Design review of the part built by this model. Coordinates are the model's own, in mm. Face numbers are marked on the shaded views. A direction names the side the tool comes from. Coordinates: 2 decimals unless noted, no trailing zeros. Order: outer loops, then holes, each group sorted by start corner. A loop starts at its lowest first (then second) coordinate and runs counter-clockwise, first axis right, second up. Notation, with made-up numbers: (38, 44) - (77, 44) arc R21 cw to (77, 66) - close; hole circle Ø5 at (84.5, 6). An arc over 180 degrees is marked (long way). Write item = value, one per line. Start each with the question number.
```python
from build123d import *

# Parameters (mm, degrees)
SKETCH1_R               = 11
SKETCH1_R_2             = 1
BOSS_EXTRUDE1_DEPTH     = 2
SKETCH2_R               = 4
CUT_EXTRUDE1_DEPTH      = 16.684387141
SKETCH4_W               = 1.5
SKETCH4_H               = 3
CUT_EXTRUDE3_DEPTH      = 4
BOSS_EXTRUDE2_START     = 20
SKETCH5_R               = 6
SKETCH5_R_2             = 4
BOSS_EXTRUDE2_DEPTH     = 20
BOSS_EXTRUDE3_START     = 20
SKETCH6_R               = 6
BOSS_EXTRUDE3_DEPTH     = 20
CUT_EXTRUDE4_DEPTH      = 5
CUT_EXTRUDE4_DEPTH_BACK = 1
SKETCH7_R               = 1
SKETCH8_R               = 2
CUT_EXTRUDE5_DEPTH      = 1


with BuildPart() as part:
    # Sketch1 → Boss-Extrude1 (new body)
    with BuildSketch(Plane(origin=(0, 0, 0), x_dir=(1, 0, 0), z_dir=(0, 1, 0))):
        with Locations(Location((0, 0, 0), (0, 0, 270))):
            Circle(SKETCH1_R)
        with Locations(Location((0, 8, 0), (0, 0, 270))):
            Circle(SKETCH1_R_2, mode=Mode.SUBTRACT)
        with Locations(Location((5.656854249, 5.656854249, 0), (0, 0, 270))):
            Circle(SKETCH1_R_2, mode=Mode.SUBTRACT)
        with Locations(Location((8, 0, 0), (0, 0, 270))):
            Circle(SKETCH1_R_2, mode=Mode.SUBTRACT)
        with Locations(Location((5.656854249, -5.656854249, 0), (0, 0, 270))):
            Circle(SKETCH1_R_2, mode=Mode.SUBTRACT)
        with Locations(Location((0, -8, 0), (0, 0, 270))):
            Circle(SKETCH1_R_2, mode=Mode.SUBTRACT)
        with Locations(Location((-5.656854249, -5.656854249, 0), (0, 0, 270))):
            Circle(SKETCH1_R_2, mode=Mode.SUBTRACT)
        with Locations(Location((-8, 0, 0), (0, 0, 270))):
            Circle(SKETCH1_R_2, mode=Mode.SUBTRACT)
        with Locations(Location((-5.656854249, 5.656854249, 0), (0, 0, 270))):
            Circle(SKETCH1_R_2, mode=Mode.SUBTRACT)
    extrude(amount=BOSS_EXTRUDE1_DEPTH)

    # Sketch2 → Cut-Extrude1 (cut, through all)
    with BuildSketch(Plane(origin=(0, 2, 0), x_dir=(1, 0, 0), z_dir=(0, 1, 0))):
        with Locations(Location((0, 0, 0), (0, 0, 270))):
            Circle(SKETCH2_R)
    extrude(amount=-CUT_EXTRUDE1_DEPTH, mode=Mode.SUBTRACT)

    # Sketch4 → Cut-Extrude3 (cut)
    with BuildSketch(Plane(origin=(0, 2, 0), x_dir=(1, 0, 0), z_dir=(0, 1, 0))):
        with Locations((0, 11)):
            Rectangle(SKETCH4_W, SKETCH4_H)
    extrude(amount=-CUT_EXTRUDE3_DEPTH, mode=Mode.SUBTRACT)

    # Sketch5 → Boss-Extrude2 (add)
    with BuildSketch(Plane(origin=(0, 2, 0), x_dir=(1, 0, 0), z_dir=(0, 1, 0)).offset(BOSS_EXTRUDE2_START)):
        with Locations(Location((0, 0, 0), (0, 0, 270))):
            Circle(SKETCH5_R)
        with Locations(Location((0, 0, 0), (0, 0, 270))):
            Circle(SKETCH5_R_2, mode=Mode.SUBTRACT)
    extrude(amount=-BOSS_EXTRUDE2_DEPTH)

    # Sketch6 → Boss-Extrude3 (add)
    with BuildSketch(Plane(origin=(0, 22, 0), x_dir=(1, 0, 0), z_dir=(0, 1, 0)).offset(BOSS_EXTRUDE3_START)):
        with Locations(Location((0, 0, 0), (0, 0, 270))):
            Circle(SKETCH6_R)
        with BuildLine():
            ThreePointArc((-0.967204218, 0.254), (-0.707472278, 0.706741095), (-0.255, 0.966941053))
            Line((-0.255, 0.966941053), (-0.255, 1.476941053))
            Line((-0.255, 1.476941053), (0.255, 1.476941053))
            Line((0.255, 1.476941053), (0.255, 0.966941053))
            ThreePointArc((0.255, 0.966941053), (0.707472278, 0.706741095), (0.967204218, 0.254))
            Line((0.967204218, 0.254), (1.475204218, 0.254))
            Line((1.475204218, 0.254), (1.475204218, -0.254))
            Line((1.475204218, -0.254), (0.967204218, -0.254))
            ThreePointArc((0.967204218, -0.254), (0.707106781, -0.707106781), (0.254, -0.967204218))
            Line((0.254, -0.967204218), (0.254, -1.475204218))
            Line((0.254, -1.475204218), (-0.254, -1.475204218))
            Line((-0.254, -1.475204218), (-0.254, -0.967204218))
            ThreePointArc((-0.254, -0.967204218), (-0.707106781, -0.707106781), (-0.967204218, -0.254))
            Line((-0.967204218, -0.254), (-1.475204218, -0.254))
            Line((-1.475204218, -0.254), (-1.475204218, 0.254))
            Line((-1.475204218, 0.254), (-0.967204218, 0.254))
        make_face(mode=Mode.SUBTRACT)
    extrude(amount=-BOSS_EXTRUDE3_DEPTH)

    # Sketch7 → Cut-Extrude4 (cut, two sides: drawn at the far end of the back side and taken through both)
    with BuildSketch(Plane.XY.offset(-CUT_EXTRUDE4_DEPTH_BACK)):
        with Locations(Location((0, 35, 0), (0, 0, 165.285661458))):
            Circle(SKETCH7_R)
    extrude(amount=CUT_EXTRUDE4_DEPTH + CUT_EXTRUDE4_DEPTH_BACK, mode=Mode.SUBTRACT)

    # Sketch8 → Cut-Extrude5 (cut)
    with BuildSketch(Plane.XY.offset(6)):
        with Locations((0, 35)):
            Circle(SKETCH8_R)
    extrude(amount=-CUT_EXTRUDE5_DEPTH, mode=Mode.SUBTRACT)


solid = part.part
```
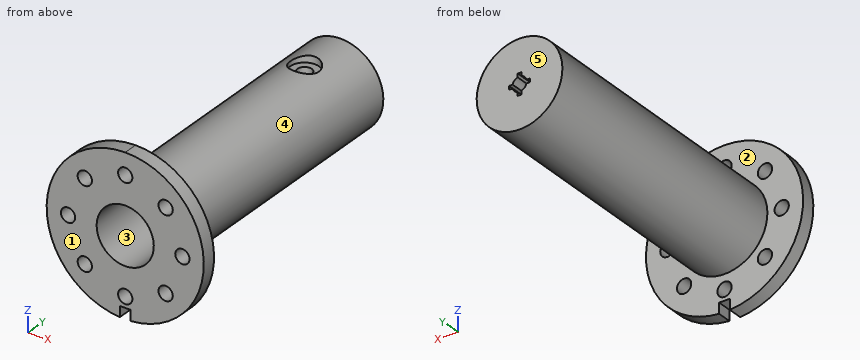
Item 1: Add section C-C on z = 2.75. Give the boundary of the cut face in (x, y), plus the area to 3 significant figures.
Item 2: Mouldability with a two-part tool opening along Z and no side actions: class the marked faces 3, 4 and 5 as +Z half, -Z half, draft (parallel to the pull), parting line (faces both ways), or undercut.
Item 3: For line 1 (X direction, y = 12.5, z = 0); line 2 (Y direction, x = -2.5, z = 8.75); line 3 (Y direction, x = -2.5, z = 1.75), list the stretches that pass through material, from the lowest coordinate up.
Item 4: Add section A-A on z = -8. Give the boundary of the cut face in (x, y).
Item 5: For P1, Ø5, axis at x = 0, z = 0, coming from the -Y side; P2, Ø8, axis at y = 27, z = 1.5, coming from the -X side; P3, Ø10, axis at y = 4.5, z = 5, coming from the -X side; P4, Ø1.6, axis at x = -8, z = 0, coming from the -Y side, all flat-tipped, find the tip position at first contact; note any pin that passes through.
Item 6: For the marked faces 1 and 2, list the 3-axis set-ups (+Z, -Z, +X, -X, +Y, -Y) from which the entire face can be reached by the end or side of a thin tool; tool diameter is ignored.
Item 7: Add section B-B on y = 28.5. Give the boundary of the cut face in (x, z) (3 decimals).
Item 8: Add section D-D on y = 15. Give the boundary of the cut face in (x, z), plus the area to 3 significant figures.
Worked out:
q1.outline = (-10.65, 0) - (-2.9, 0) - (-2.9, 22) - (2.9, 22) - (2.9, 0) - (10.65, 0) - (10.65, 2) - (5.33, 2) - (5.33, 42) - (-5.33, 42) - (-5.33, 2) - (-10.65, 2) - close; hole circle Ø2 at (0, 35)
q1.area = 338 mm2
q2.face_3 = undercut
q2.face_4 = parting line
q2.face_5 = draft
q3.line_1 = -6 to -4, 4 to 6
q3.line_2 = 0 to 2
q3.line_3 = 22 to 42
q4.outline = (-7.55, 0) - (-1, 0) - (-1, 2) - (-7.55, 2) - close; (1, 0) - (7.55, 0) - (7.55, 2) - (1, 2) - close
q5.P1 = 22
q5.P2 = -6
q5.P3 = -10.98
q5.P4 = through
q6.face_1 = +Z, -Z, +X, -X, -Y
q6.face_2 = +Y
q7.outline = circle Ø12 at (0, 0); hole (-1.475, -0.254) - (-0.967, -0.254) arc R1 ccw to (-0.255, -0.967) - (-0.255, -1.477) - (0.255, -1.477) - (0.255, -0.967) arc R1 ccw to (0.967, -0.254) - (1.475, -0.254) - (1.475, 0.254) - (0.967, 0.254) arc R1 ccw to (0.254, 0.967) - (0.254, 1.475) - (-0.254, 1.475) - (-0.254, 0.967) arc R1 ccw to (-0.967, 0.254) - (-1.475, 0.254) - close
q8.outline = circle Ø12 at (0, 0); hole circle Ø8 at (0, 0)
q8.area = 62.8 mm2
